from build123d import *

# Parameters (mm, degrees)
F0_W      = 103.75
F0_H      = 64.5
F1_DEPTH  = 2.2
F2_T      = -1.9
F3_W      = 26.5
F3_H      = 15
F4_DEPTH  = 12.7
F5_R      = 2
F6_R      = 2
F7_W      = 4.9
F7_H      = 60.7
F8_DEPTH  = 2.5
F9_W      = 4.9
F9_H      = 60.7
F10_DEPTH = 2.5
F12_DEPTH = 4.4


with BuildPart() as f1:
    # F0 (on Top) → F1 (new body, symmetric)
    with BuildSketch(Plane.XY):
        Rectangle(F0_W, F0_H)
    extrude(amount=F1_DEPTH, both=True)

    # F2
    f2_openings = [f1.faces().sort_by_distance(p)[0] for p in [
        (0, 0, 2.2),
    ]]
    offset(amount=F2_T, openings=f2_openings)

    # F3 (on Top) → F4 (cut, symmetric)
    with BuildSketch(Plane.XY):
        Rectangle(F3_W, F3_H)
    extrude(amount=F4_DEPTH, both=True, mode=Mode.SUBTRACT)

    # F5
    f5_edges = [f1.edges().sort_by_distance(p)[0] for p in [
        (-51.875, 32.25, 0),
    ]]
    fillet(f5_edges, radius=F5_R)

    # F6
    f6_edges = [f1.edges().sort_by_distance(p)[0] for p in [
        (-51.875, -32.25, 0),
        (51.875, -32.25, 0),
        (51.875, 32.25, 0),
    ]]
    fillet(f6_edges, radius=F6_R)

    # F7 (on face) → F8 (join)
    with BuildSketch(Plane.XY.offset(-0.3)):
        with Locations((-47.525, 0)):
            Rectangle(F7_W, F7_H)
    extrude(amount=F8_DEPTH)

    # F9 (on face) → F10 (join)
    with BuildSketch(Plane.XY.offset(-0.3)):
        with Locations((47.525, 0)):
            Rectangle(F9_W, F9_H)
    extrude(amount=F10_DEPTH)

    # F11 (on face) → F12 (cut)
    with BuildSketch(Plane.XY.offset(2.2)):
        with BuildLine():
            ThreePointArc((-48.475, 29.75), (-49.853858, 26.421142), (-46.525, 27.8))
            ThreePointArc((-46.525, 27.8), (-47.096142, 29.178858), (-48.475, 29.75))
        make_face()
        with BuildLine():
            ThreePointArc((48.474999, 29.75), (47.096141, 26.421142), (50.424999, 27.8))
            ThreePointArc((50.424999, 27.8), (49.853858, 29.178858), (48.474999, 29.75))
        make_face()
        with BuildLine():
            ThreePointArc((-48.472498, -29.75), (-47.09364, -29.178858), (-46.522498, -27.8))
            ThreePointArc((-46.522498, -27.8), (-49.851357, -26.421142), (-48.472498, -29.75))
        make_face()
        with BuildLine():
            ThreePointArc((48.477501, -29.75), (49.856359, -29.178858), (50.427501, -27.8))
            ThreePointArc((50.427501, -27.8), (47.098643, -26.421142), (48.477501, -29.75))
        make_face()
    extrude(amount=-F12_DEPTH, mode=Mode.SUBTRACT)


solid = f1.part
Source: CAD feature listing. Evaluate the final solid. Frame: model axes, mm. A direction names the side the tool comes from. Round coordinates to 2 decimals unless told otherwise and drop trailing zeros. Loops run counter-clockwise (first coordinate to the right, second up) from the corner with the lowest first, then second, coordinate; pieces in that order, holes last. Notation, with made-up numbers: (-32, 37.5) - (7, 37.5) arc R25 ccw to (7, 50.5) - close; hole circle Ø8 at (58, 67.5). An arc over 180 degrees is marked (long way). Write item = value, one per line. Start each with the question number.
(1) Section query A-A, the plane x = -5. Output: boundary loops of the cut face in (y, z), plus the area to 3 significant figures.
(2) Section query D-D, the plane x = 24.5. Output: boundary loops of the cut face in (y, z).
(3) Section query B-B, the plane z = 1.35. State how many separate pieces and enclosed holes the cut face has, plus the area to 3 significant figures.
(4) Set-up query: faces 5 (the face through (-51.875, 0, 0)), 6 (the face through (-1, 14, -0.3)), 7 (the face through (-13.25, 0, -1)). Return all of +Z, -Z, +X, -X, +Y, -Y with unobstructed straight access to the full face (end or side cutting, diameter ignored); none if empty.
(5) Section query C-C, the plane y = 23.5. Output: boundary loops of the cut face in (x, z) (3 decimals).
(6) Pull-direction query (Y, two-part tool) for faces 1 (the face through (-1, 32.25, 0)), 2 (the face through (-1, -32.25, 0)), 3 (the face through (51.875, 0, 0)), 4 (the face through (-1, -30.35, 1)); classes: +Y half, -Y half, draft (parallel to the pull), parting line (faces both ways), or undercut.
(7) Ray query, line 1 along X through (y, z) = (27.8, 1.3) (3 decimals); line 2 along X through (y, z) = (-27.5, -0.7) (3 decimals); line 3 along X through (y, z) = (27.8, -1.3) (3 decimals). Return the intervals inside material, ascending. Write a range as from..to.
(8) Pin query (flat end, axial travel): pin 1 (4 mm diameter, centred on x = -32.5, y = 6, fed in from +Z); pin 2 (6 mm diameter, centred on x = 48.475, y = 27.8, fed in from +Z). Return the tip coordinate at first contact, or that it passes through.
Conclusion:
q1.outline = (-32.25, -2.2) - (-7.5, -2.2) - (-7.5, -0.3) - (-30.35, -0.3) - (-30.35, 2.2) - (-32.25, 2.2) - close; (7.5, -2.2) - (32.25, -2.2) - (32.25, 2.2) - (30.35, 2.2) - (30.35, -0.3) - (7.5, -0.3) - close
q1.area = 104 mm2
q2.outline = (-32.25, -2.2) - (32.25, -2.2) - (32.25, 2.2) - (30.35, 2.2) - (30.35, -0.3) - (-30.35, -0.3) - (-30.35, 2.2) - (-32.25, 2.2) - close
q3.separate_pieces = 1
q3.enclosed_holes = 5
q3.area = 1,170 mm2
q4.face_5 = +Z, -Z, -X, +Y, -Y
q4.face_6 = +Z
q4.face_7 = +Z, -Z
q5.outline = (-51.875, -2.2) - (51.875, -2.2) - (51.875, 2.2) - (45.075, 2.2) - (45.075, -0.3) - (-45.075, -0.3) - (-45.075, 2.2) - (-51.875, 2.2) - close
q6.face_1 = +Y half
q6.face_2 = -Y half
q6.face_3 = draft
q6.face_4 = undercut
q7.line_1 = -51.875..-50.425, -46.525..-45.075, 45.075..46.525, 50.425..51.875
q7.line_2 = -51.875..-50.399, -46.546..46.551, 50.404..51.875
q7.line_3 = -51.875..-50.425, -46.525..46.525, 50.425..51.875
q8.pin_1 = -0.3
q8.pin_2 = 2.2
